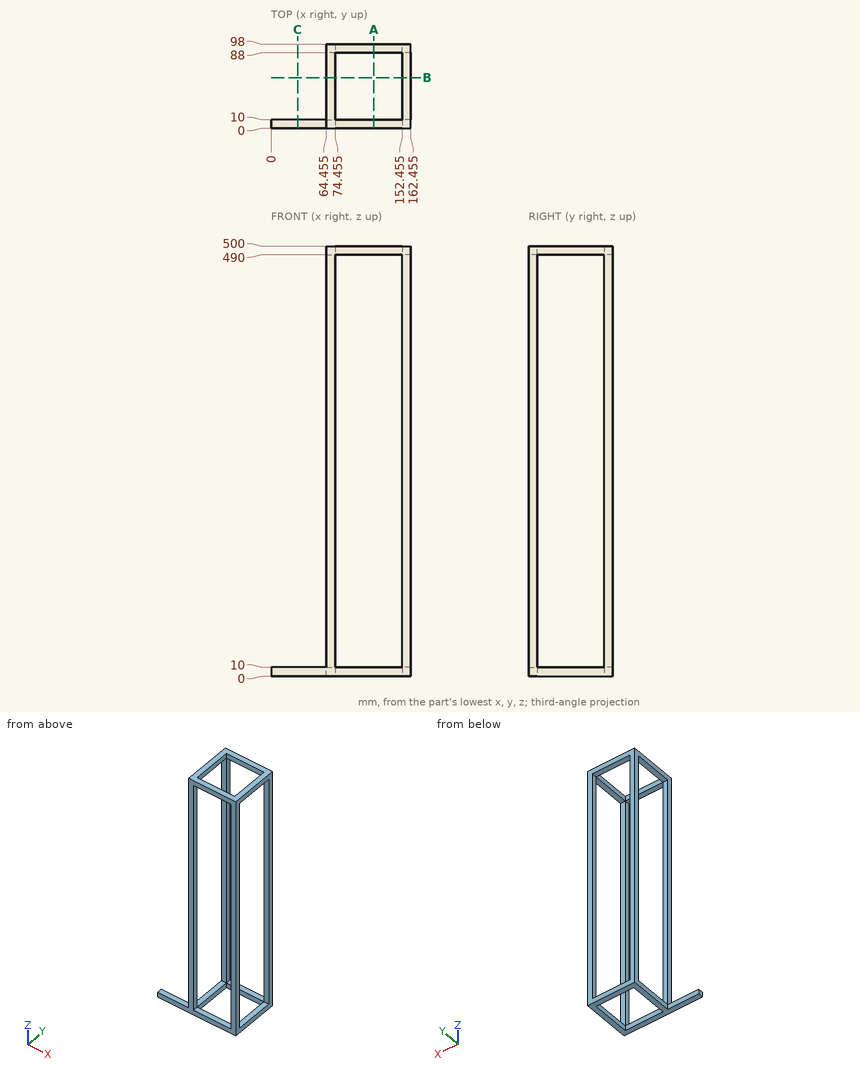
Input: dimensioned drawing with shaded views. Units: mm. Origin: part minimum x, y, z. Round coordinates to 2 decimals unless told otherwise and drop trailing zeros. Order: outer loops, then holes, each group sorted by start corner. A loop starts at its lowest first (then second) coordinate and runs counter-clockwise, first axis right, second up. Notation, with made-up numbers: (16, 56) - (33, 56) arc R17 ccw to (33, 62) - close; hole circle Ø7 at (30.25, -27.5). An arc over 180 degrees is marked (long way). Write item = value, one per line. Start each with the question number.
Q1. Ray query, line 1 (Z direction, x = 69, y = 85.5); line 2 (X direction, y = 4, z = 99) (3 decimals); line 3 (Z direction, x = 42, y = 8). Return the intervals inside material, ascending. Write a range as from..to.
Q2. Cut plane A-A on x = 119.5. Return the cut outline in (y, z).
Q3. Pin query (flat end, axial travel): pin 1 (5 mm diameter, centred on y = 64.5, z = 494.5, fed in from -X) (3 decimals); pin 2 (3 mm diameter, centred on x = 30.5, y = 5.5, fed in from +Z). Return the tip coordinate at first contact, or that it passes through.
Q4. Cut plane C-C on x = 31. Return the cut outline in (y, z).
Q5. Cut plane B-B on y = 59. Return the cut outline in (x, z) (3 decimals), and give its area (3 significant figures).
Outcome:
q1.line_1 = 0..10, 490..500
q1.line_2 = 64.455..74.455, 152.455..162.455
q1.line_3 = 0..10
q2.outline = (0, 0) - (10, 0) - (10, 10) - (0, 10) - close; (0, 490) - (10, 490) - (10, 500) - (0, 500) - close; (88, 0) - (98, 0) - (98, 10) - (88, 10) - close; (88, 490) - (98, 490) - (98, 500) - (88, 500) - close
q3.pin_1 = 64.455
q3.pin_2 = 10
q4.outline = (0, 0) - (10, 0) - (10, 10) - (0, 10) - close
q5.outline = (64.455, 0) - (74.455, 0) - (74.455, 10) - (64.455, 10) - close; (64.455, 490) - (74.455, 490) - (74.455, 500) - (64.455, 500) - close; (152.455, 0) - (162.455, 0) - (162.455, 10) - (152.455, 10) - close; (152.455, 490) - (162.455, 490) - (162.455, 500) - (152.455, 500) - close
q5.area = 400 mm^2
